Source: CAD feature listing. Evaluate the final solid. Frame: model axes, mm. Face numbers are marked on the shaded views. A direction names the side the tool comes from. Give positions to 0.01 mm unless a question says otherwise; leave off trailing zeros. Loops run counter-clockwise (first coordinate to the right, second up) from the corner with the lowest first, then second, coordinate; pieces in that order, holes last.
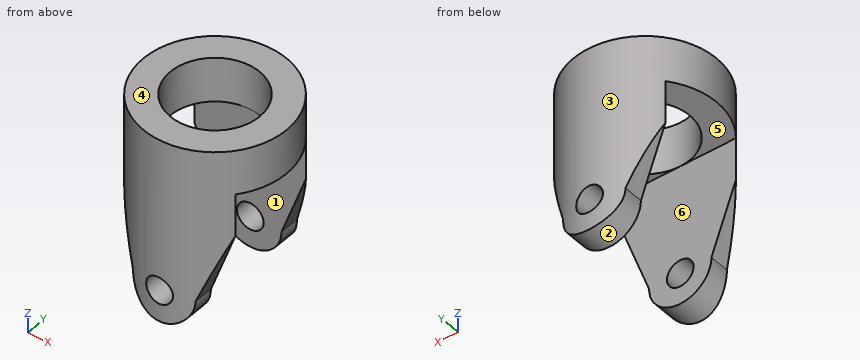
```python
from build123d import *

# Parameters (mm, degrees)
SKETCH1_R               = 8
SKETCH1_R_2             = 5
BOSS_EXTRUDE1_DEPTH     = 20.75
SKETCH2_R               = 1.5
CUT_EXTRUDE1_DEPTH      = 9
CUT_EXTRUDE1_DEPTH_BACK = 9
SKETCH4_W               = 15.75
SKETCH4_H               = 10
CUT_EXTRUDE2_DEPTH      = 9.0000001
CUT_EXTRUDE2_DEPTH_BACK = 9.0000001


with BuildPart() as part:
    # Sketch1 → Boss-Extrude1 (new body)
    with BuildSketch(Plane.XY):
        Circle(SKETCH1_R)
        Circle(SKETCH1_R_2, mode=Mode.SUBTRACT)
    extrude(amount=BOSS_EXTRUDE1_DEPTH)

    # Sketch2 → Cut-Extrude1 (cut, two sides)
    with BuildSketch(Plane(origin=(0, 0, 0), x_dir=(1, 0, 0), z_dir=(0, 1, 0))) as cut_extrude1_sk:
        with Locations((0, -3.5)):
            Circle(SKETCH2_R)
        with BuildLine():
            Line((-8, -15.75), (-8, 2.25))
            Line((-8, 2.25), (8, 2.25))
            Line((8, 2.25), (8, -15.75))
            Line((8, -15.75), (3.5, -3.5))
            ThreePointArc((3.5, -3.5), (0, 0), (-3.5, -3.5))
            Line((-3.5, -3.5), (-8, -15.75))
        make_face()
    extrude(amount=CUT_EXTRUDE1_DEPTH, mode=Mode.SUBTRACT)
    extrude(cut_extrude1_sk.sketch, amount=-CUT_EXTRUDE1_DEPTH_BACK, mode=Mode.SUBTRACT)

    # Sketch4 → Cut-Extrude2 (cut, two sides)
    with BuildSketch(Plane(origin=(0, 0, 0), x_dir=(0, 0, -1), z_dir=(1, 0, 0))) as cut_extrude2_sk:
        with Locations((-7.875, 0)):
            Rectangle(SKETCH4_W, SKETCH4_H)
    extrude(amount=CUT_EXTRUDE2_DEPTH, mode=Mode.SUBTRACT)
    extrude(cut_extrude2_sk.sketch, amount=-CUT_EXTRUDE2_DEPTH_BACK, mode=Mode.SUBTRACT)


solid = part.part
```
(1) Section A-A, the plane y = 0. Return the cut outline in (x, z), then the cut area to 3 significant figures.
A:
outline: (-8, 15.75) - (-5, 15.75) - (-5, 20.75) - (-8, 20.75) - close; (5, 15.75) - (8, 15.75) - (8, 20.75) - (5, 20.75) - close
area: 30.0 mm2
(2) Section C-C, the plane z = 15.25. Return the cut outline in (x, y) (3 decimals).
A:
outline: (-6.245, -5) arc R8 ccw to (6.245, -5) - close; (-6.245, 5) - (6.245, 5) arc R8 ccw to start
(3) Section B-B, the plane x = -3.75. Return the cut outline in (y, z), then the cut area to 3 significant figures.
A:
outline: (-7.07, 4.18) - (-5, 4.18) - (-5, 15.75) - (-3.31, 15.75) - (-3.31, 20.75) - (-7.07, 20.75) - close; (3.31, 15.75) - (5, 15.75) - (5, 4.18) - (7.07, 4.18) - (7.07, 20.75) - (3.31, 20.75) - close
area: 85.4 mm2
(4) Section D-D, the plane y = -5.75. Return the cut outline in (x, z).
A:
outline: (-5.56, 9.11) - (-3.5, 3.5) arc R3.5 ccw to (3.5, 3.5) - (5.56, 9.11) - (5.56, 20.75) - (-5.56, 20.75) - close; hole circle Ø3 at (0, 3.5)
(5) Reachability of the marked faces 1 and 2 from +Z, -Z, +X, -X, +Y, -Y: full face, straight path, thin tool, end or side. Return the list, or none.
A:
face 1: -Z, +X, -X
face 2: -Z, +Y, -Y
(6) Ray query, line 1 along X through (y, z) = (0, 17.15); line 2 along X through (y, z) = (-5.65, 3.5). Return the intervals inside material, ascending.
A:
line 1: x = -8 to -5, 5 to 8
line 2: x = -3.5 to -1.5, 1.5 to 3.5
(7) Mould query, pull axis Y, two halves, no side actions, for the marked faces 3, 4, 5 and 6. Classes: pulls with the +Y half, pulls with the -Y half, needs draft (parallel to the pull), parting line crosses it, or undercut.
A:
face 3: parting line crosses it
face 4: needs draft
face 5: undercut
face 6: undercut
(8) First-contact query: pin 1 (8 mm diameter, centred on x = 5.5, z = 10.5, fed in from -Y); pin 2 (2 mm diameter, centred on x = 3.5, z = 5.5, fed in from +Y); pin 3 (1.5 mm diameter, centred on y = 6, z = 16.5, fed in from -X). Flat tips, straight axial feed; report the tip coordinate or a pass-through.
A:
pin 1: stops at y = -7.86
pin 2: stops at y = 7.6
pin 3: stops at x = -6.04
